```python
from build123d import *

# Parameters (mm, degrees)
BOSS_EXTRUDE1_DEPTH = 6.35
CUT_EXTRUDE2_DEPTH  = 468.016490608
FILLET1_R           = 12.7


with BuildPart() as part:
    # Sketch1 → Boss-Extrude1 (new body)
    with BuildSketch(Plane(origin=(0, 0, 0), x_dir=(1, 0, 0), z_dir=(0, 1, 0))):
        Polygon((-330.2, 152.4), (-330.2, -152.4), (-241.3, -152.4), (-152.4, -241.3), (-152.4, -330.2), (152.4, -330.2), (152.4, -241.3), (241.3, -152.4), (330.2, -152.4), (330.2, 152.4), (241.3, 152.4), (152.4, 241.3), (152.4, 330.2), (-152.4, 330.2), (-152.4, 241.3), (-241.3, 152.4), align=None)
    extrude(amount=BOSS_EXTRUDE1_DEPTH)

    # Sketch3 → Cut-Extrude2 (cut, through all)
    with BuildSketch(Plane(origin=(0, 6.35, 0), x_dir=(1, 0, 0), z_dir=(0, 1, 0))):
        with BuildLine():
            Line((69.85, 330.2), (-38.1, 330.2))
            Line((-38.1, 330.2), (-38.1, 165.1))
            ThreePointArc((-38.1, 165.1), (-34.380256121, 156.119743879), (-25.4, 152.4))
            Line((-25.4, 152.4), (57.15, 152.4))
            ThreePointArc((57.15, 152.4), (66.130256121, 156.119743879), (69.85, 165.1))
            Line((69.85, 165.1), (69.85, 330.2))
        make_face()
        with BuildLine():
            Line((69.85, -330.2), (-38.1, -330.2))
            Line((-38.1, -330.2), (-38.1, -165.1))
            ThreePointArc((-38.1, -165.1), (-34.380256121, -156.119743879), (-25.4, -152.4))
            Line((-25.4, -152.4), (57.15, -152.4))
            ThreePointArc((57.15, -152.4), (66.130256121, -156.119743879), (69.85, -165.1))
            Line((69.85, -165.1), (69.85, -330.2))
        make_face()
    extrude(amount=-CUT_EXTRUDE2_DEPTH, mode=Mode.SUBTRACT)

    # Fillet1
    fillet1_edges = [part.edges().sort_by_distance(p)[0] for p in [
        (152.4, 3.175, 241.3),
        (-152.4, 3.175, 241.3),
        (-241.3, 3.175, 152.4),
        (-241.3, 3.175, -152.4),
        (-152.4, 3.175, -241.3),
        (152.4, 3.175, -241.3),
        (241.3, 3.175, -152.4),
        (241.3, 3.175, 152.4),
    ]]
    fillet(fillet1_edges, radius=FILLET1_R)


solid = part.part
```
Model file for the job. Use its own axes, mm. Coordinates: 2 decimals unless noted, no trailing zeros. Order: outer loops, then holes, each group sorted by start corner. A loop starts at its lowest first (then second) coordinate and runs counter-clockwise, first axis right, second up. Notation, with made-up numbers: (-37.75, -12) -> (1.25, -12) arc R13 ccw to (1.25, -5) -> close; hole circle Ø10 at (32.5, 62). An arc over 180 degrees is marked (long way). Return JSON: item names as keys, results as strings.
Item 1: Slice it at A-A (z = 173.5). Write the cut outline in (x, y).
Model answer:
{"outline": "(-220.2, 0) -> (-38.1, 0) -> (-38.1, 6.35) -> (-220.2, 6.35) -> close; (69.85, 0) -> (220.2, 0) -> (220.2, 6.35) -> (69.85, 6.35) -> close"}
Item 2: Slice it at B-B (x = 177). Write the cut outline in (y, z), then the cut area to 3 significant figures.
Model answer:
{"outline": "(0, -216.7) -> (6.35, -216.7) -> (6.35, 216.7) -> (0, 216.7) -> close", "area": "2,750 mm²"}
Item 3: Slice it at C-C (x = -197). Write the cut outline in (y, z), then the cut area to 3 significant figures.
Model answer:
{"outline": "(0, -196.7) -> (6.35, -196.7) -> (6.35, 196.7) -> (0, 196.7) -> close", "area": "2,500 mm²"}
Item 4: Pin check, flat tips, straight feed: P1, Ø1.9, axis at x = -272.5, y = 2, coming from the +Z side; P2, Ø3, axis at x = -297.5, y = 3.5, coming from the -Z side; P3, Ø4, axis at x = 57.5, z = 7, coming from the -Y side; P4, Ø1.9, axis at y = 4.5, z = 221, coming from the -X side. Stop position of each tip, or through.
Model answer:
{"P1": "stops at z = 152.4", "P2": "stops at z = -152.4", "P3": "stops at y = 0", "P4": "stops at x = -173.65"}
Item 5: Wall check: line 1 along X through (y, z) = (5.5, -263.5); line 2 along X through (y, z) = (4, 245); line 3 along Z through (x, y) = (-26.5, 4.5). Give the ranges that are in metal, low to high. Write a range as from..to.
Model answer:
{"line 1": "x = -152.4..-38.1, 69.85..152.4", "line 2": "x = -152.5..-38.1, 69.85..152.5", "line 3": "z = -152.45..152.45"}
